Can you work these out from the model? Positions are in its coordinate system, mm. Round coordinates to 2 decimals unless told otherwise and drop trailing zeros. Write each loop counter-clockwise with the first axis right and the second up, starting at its lowest first coordinate (ties: lowest second). Pieces come first, ordered by that corner, then holes. Notation, with made-up numbers: (82, 44.25) -> (113, 44.25) arc R18 ccw to (113, 50.25) -> close; hole circle Ø9 at (32.25, 64.5). An arc over 180 degrees is marked (long way). Write item = value, one per line. Start each with the question number.
1) Imagine slicing it at A-A, the plane z = 72.5. Please give me the cut outline in (x, y), then the cut area to 3 significant figures.
2) Imagine slicing it at B-B, the plane x = -26.5. State how many separate pieces and enclosed holes the cut face has, then the cut area to 3 significant figures.
3) I'm going to push flat-ended pins straight in: pin 1 (1 mm diameter, centred on y = -13.5, z = 106, fed in from -X); pin 2 (5 mm diameter, centred on y = 10.5, z = 34.5, fed in from -X); pin 3 (1.5 mm diameter, centred on x = 0, z = 77, fed in from +Y); pin 4 (1.1 mm diameter, centred on y = 0, z = 0.5, fed in from +X). Where does each tip first touch, or does it pass through?
4) Thinking about a two-plate mould opening in Z: for faces 1 (the face through (24.273, -0.032, 92.874)), 2 (the face through (2, -20, 20)), 3 (the face through (2.219, 17.639, 24.003)), which applies, +Z half, -Z half, draft (parallel to the pull), parting line (faces both ways), or undercut?
5) If I drill on line 1 (X direction, y = -11, z = 15.5); line 2 (X direction, y = -31, z = 42.5); line 3 (Z direction, x = 12, y = 28), over which ranges is the centre line in solid material (lowest first)?
from build123d import *

# Parameters (mm, degrees)
F1_DEPTH = 4.5
F5_DEPTH = 2.25
F7_DEPTH = 12.5


with BuildPart() as f1:
    # F0 (on Right) → F1 (new body)
    with BuildSketch(Plane.YZ):
        Polygon((-40, 40), (0, 0), (40, 40), (0, 150), align=None)
        Polygon((-34.7915337519, 41.1554947826), (0, 136.8322126004), (34.7915337519, 41.1554947826), (0, 6.3639610307), align=None, mode=Mode.SUBTRACT)
    extrude(amount=F1_DEPTH)

    # F4 (on Front) → F5 (join, symmetric)
    with BuildSketch(Plane.XZ):
        Polygon((-40, 40), (0, 0), (0, 6.3639610307), (-34.7915337519, 41.1554947826), (0, 136.8322126004), (0, 150), align=None)
        Polygon((38.2915337519, 41.1554947826), (3.5, 6.3639610307), (3.5, 0), (43.5, 40), (3.5, 150), (3.5, 136.8322126004), align=None)
    extrude(amount=F5_DEPTH, both=True)

    # F6 (on offset) → F7 (cut, symmetric)
    with BuildSketch(Plane.YZ.offset(1.75)):
        Polygon((-46.8705444882, 150), (-40, 40), (0, 150), align=None)
        Polygon((46.8705444882, 150), (0, 150), (40, 40), align=None)
        Polygon((0, 0), (-40, 40), (-40, 0), align=None)
        Polygon((40, 40), (0, 0), (40, 0), align=None)
    extrude(amount=F7_DEPTH, both=True, mode=Mode.SUBTRACT)

    # F8 (on face) → F10 section 0
    with BuildSketch(Plane.YZ.offset(4.5)):
        Polygon((-38.6330277477, 43.759173694), (-40, 40), (-37.1715728753, 37.1715728753), (-34.7915337519, 41.1554947826), align=None)
    # F9 (on face) → F10 section 1
    with BuildSketch(Plane.XZ.offset(2.25)):
        Polygon((40.6715728753, 37.1715728753), (43.5, 40), (42.1330277477, 43.759173694), (38.2915337519, 41.1554947826), align=None)
    loft()

    # F11 (on face) → F13 section 0
    with BuildSketch(Plane(origin=(0, 2.25, 0), x_dir=(-1, 0, 0), z_dir=(0, 1, 0))):
        Polygon((-42.1330277477, 43.759173694), (-43.5, 40), (-40.6715728753, 37.1715728753), (-38.2915337519, 41.1554947826), align=None)
    # F12 (on face) → F13 section 1
    with BuildSketch(Plane.YZ.offset(4.5)):
        Polygon((37.1715728753, 37.1715728753), (40, 40), (38.6330277477, 43.759173694), (34.7915337519, 41.1554947826), align=None)
    loft()

    # F15 (on face) → F16 section 0
    with BuildSketch(Plane(origin=(0, 2.25, 0), x_dir=(-1, 0, 0), z_dir=(0, 1, 0))):
        Polygon((37.1715728753, 37.1715728753), (40, 40), (38.6330277477, 43.759173694), (34.7915337519, 41.1554947826), align=None)
    # F14 (on face) → F16 section 1
    with BuildSketch(Plane(origin=(0, 0, 0), x_dir=(0, -1, 0), z_dir=(-1, 0, 0))):
        Polygon((-38.6330277477, 43.759173694), (-40, 40), (-37.1715728753, 37.1715728753), (-34.7915337519, 41.1554947826), align=None)
    loft()

    # F17 (on face) → F19 section 0
    with BuildSketch(Plane.XZ.offset(2.25)):
        Polygon((-38.6330277477, 43.759173694), (-40, 40), (-37.1715728753, 37.1715728753), (-34.7915337519, 41.1554947826), align=None)
    # F18 (on face) → F19 section 1
    with BuildSketch(Plane(origin=(0, 0, 0), x_dir=(0, -1, 0), z_dir=(-1, 0, 0))):
        Polygon((37.1715728753, 37.1715728753), (40, 40), (38.6330277477, 43.759173694), (34.7915337519, 41.1554947826), align=None)
    loft()


solid = f1.part
Reported:
q1.outline = (-28.18, -2.25) -> (-23.39, -2.25) -> (-23.39, 2.25) -> (-28.18, 2.25) -> close; (0, -28.18) -> (4.5, -28.18) -> (4.5, -23.39) -> (0, -23.39) -> close; (0, 23.39) -> (4.5, 23.39) -> (4.5, 28.18) -> (0, 28.18) -> close; (26.89, -2.25) -> (31.68, -2.25) -> (31.68, 2.25) -> (26.89, 2.25) -> close
q1.area = 86.2 mm²
q2.separate_pieces = 4
q2.enclosed_holes = 0
q2.area = 122 mm²
q3.pin_1 = 0
q3.pin_2 = through
q3.pin_3 = 26.82
q3.pin_4 = 4.55
q4.face_1 = +Z half
q4.face_2 = -Z half
q4.face_3 = undercut
q5.line_1 = 0 to 4.5
q5.line_2 = -8.59 to -6.15, 10.48 to 12.87
q5.line_3 = 40.43 to 41.45
